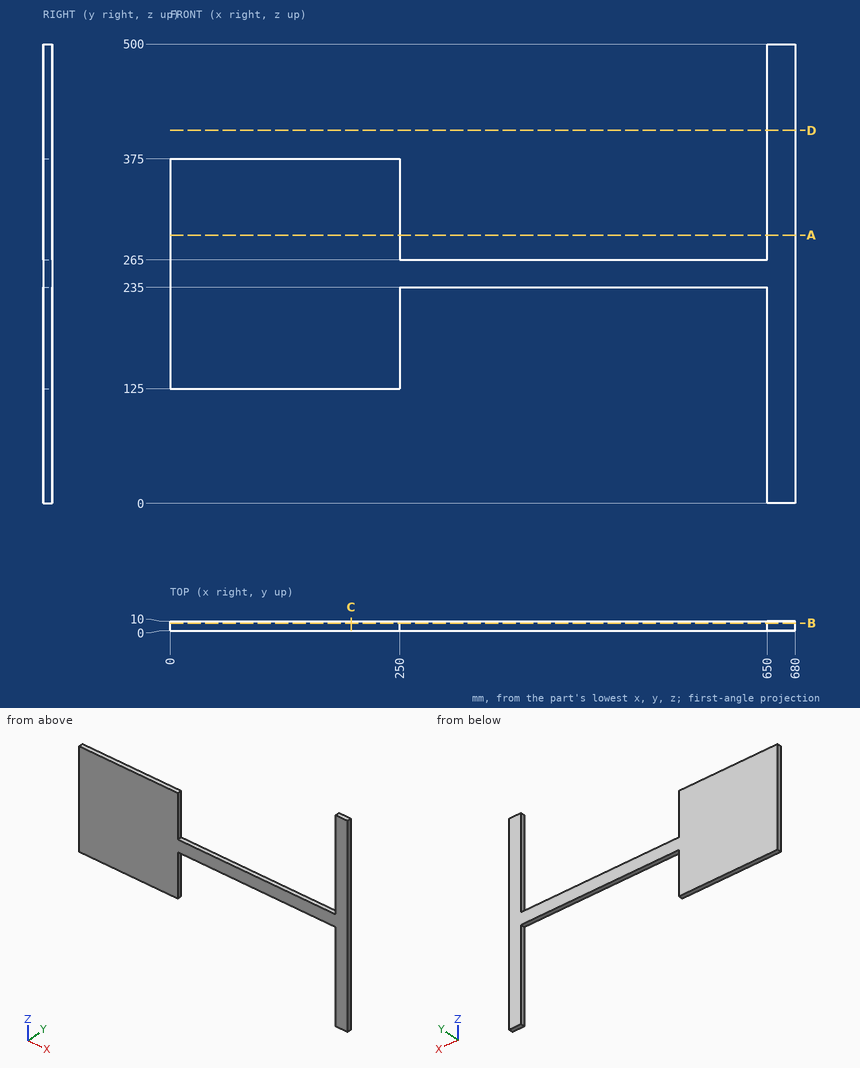
Source: three-view drawing plus pictorial views. Frame: mm from the lowest corner of the part. Give positions to 0.01 mm unless a question says otherwise; leave off trailing zeros. Order: outer loops, then holes, each group sorted by start corner. A loop starts at its lowest first (then second) coordinate and runs counter-clockwise, first axis right, second up. Notation, with made-up numbers: M 54,51.25 L 83,51.25 A26 cw 83,90.25 Z; hole C 71,80 d6. An arc over 180 degrees is marked long. Return JSON: item names as keys, results as strings.
1) Section query D-D on z = 406. Output: boundary loops of the cut face in (x, y), and give its area (3 significant figures).
Taken from the geometry:
{"outline": "M 650,0 L 680,0 L 680,10 L 650,10 Z", "area": "300 mm2"}
2) Section query B-B on y = 8.25. Output: boundary loops of the cut face in (x, z), and give its area (3 significant figures).
Taken from the geometry:
{"outline": "M 0,125 L 250,125 L 250,235 L 650,235 L 650,0 L 680,0 L 680,500 L 650,500 L 650,265 L 250,265 L 250,375 L 0,375 Z", "area": "89,500 mm2"}
3) Section query C-C on x = 197. Output: boundary loops of the cut face in (y, z), and give its area (3 significant figures).
Taken from the geometry:
{"outline": "M 0,125 L 10,125 L 10,375 L 0,375 Z", "area": "2,500 mm2"}
4) Contact query for flat-ended pins moving along their axis: pin 1 (1.5 mm diameter, centred on x = 287, y = 3.5, fed in from -Z); pin 2 (3 mm diameter, centred on x = 168.5, y = 7, fed in from +Z); pin 3 (6 mm diameter, centred on x = 584, y = 6, fed in from +Z); pin 4 (5 mm diameter, centred on y = 4.5, z = 372.5, fed in from -X). Output: stop coordinate, or through.
Taken from the geometry:
{"pin 1": "stops at z = 235", "pin 2": "stops at z = 375", "pin 3": "stops at z = 265", "pin 4": "stops at x = 0"}
5) Line query: L1, parallel to X at y = 7.5, z = 168; L2, parallel to Z at x = 430.5, y = 1.25; L3, parallel to X at y = 8.5, z = 393. Output: solid intervals per line, ascending. Write a range as [from, to].
Taken from the geometry:
{"L1": "x = [0, 250], [650, 680]", "L2": "z = [235, 265]", "L3": "x = [650, 680]"}
6) Section query A-A on z = 292. Output: boundary loops of the cut face in (x, y), and give its area (3 significant figures).
Taken from the geometry:
{"outline": "M 0,0 L 250,0 L 250,10 L 0,10 Z; M 650,0 L 680,0 L 680,10 L 650,10 Z", "area": "2,800 mm2"}
